The listing builds one solid part. Answer for the finished solid, in the listing's coordinates (mm). Face numbers are marked on the shaded views. A direction names the side the tool comes from. Give positions to 0.01 mm unless a question says otherwise; leave off trailing zeros. Write each loop counter-clockwise with the first axis right and the second up, starting at its lowest first coordinate (ties: lowest second). Pieces come first, ordered by that corner, then holes. Notation, with made-up numbers: M -7,-3 L 25,-3 A25 ccw 25,13 Z; hole C 12,28 d6. An arc over 180 degrees is marked long. Return JSON: item names as keys, results as strings.
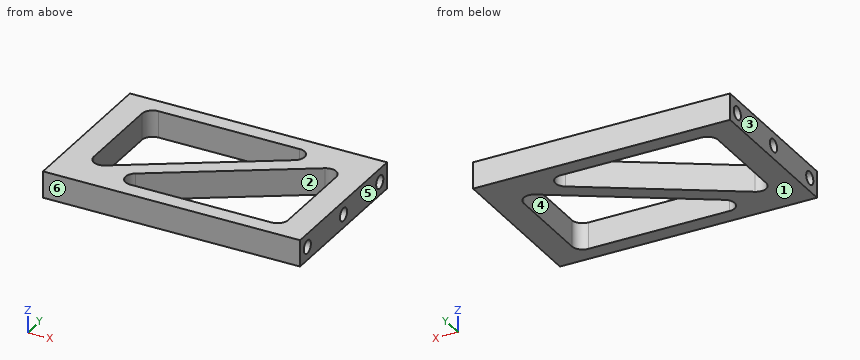
Autodesk Inventor part; units mm, degrees
ref_plane "YZ Plane" through (0, 0, 0) normal (1, 0, 0) x (0, 1, 0)
ref_plane "XZ Plane" through (0, 0, 0) normal (0, 1, 0) x (-1, 0, 0)
ref_plane "XY Plane" through (0, 0, 0) normal (0, 0, 1) x (1, 0, 0)
sketch "スケッチ1" plane through (0, 0, 0) normal (0, 0, 1) x (1, 0, 0)
  line L0 (-24.25, 15) -> (24.25, 15)
  line L1 (24.25, 15) -> (24.25, -15)
  line L2 (24.25, -15) -> (-24.25, -15)
  line L3 (-24.25, -15) -> (-24.25, 15)
  line L4 (-19.25, 12) -> (19.25, 12) construction
  line L5 (19.25, 12) -> (19.25, -12) construction
  line L6 (19.25, -12) -> (-19.25, -12) construction
  line L7 (-19.25, -12) -> (-19.25, 12) construction
  line L8 (19.25, 12) -> (-19.25, -12) construction
  line L9 (-19.25, -10.2324) -> (-19.25, 12)
  line L10 (-19.25, 12) -> (16.4145, 12)
  line L11 (16.4145, 12) -> (-19.25, -10.2324)
  line L12 (-16.4145, -12) -> (19.25, -12)
  line L13 (19.25, -12) -> (19.25, 10.2324)
  line L14 (19.25, 10.2324) -> (-16.4145, -12)
  line L15 (-24.25, 12.5) -> (24.25, 12.5) construction
  line L16 (24.25, -12.5) -> (-24.25, -12.5) construction
  line L17 (24.25, 12.5) -> (24.25, -12.5) construction
  point P0 (0, 0)
  point P1 (0, 12)
  point P2 (0, 15)
  point P3 (19.25, 0)
  point P4 (24.25, 0)
  dimension "d0" = 5
  dimension "d1" = 3
  dimension "d2" = 1.5
  dimension "d3" = 25
  dimension "d4" = 2.5
  dimension "d16" = 48.5
extrude "押し出し1" add sketch "スケッチ1" along normal blind 5
sketch "スケッチ2" plane through (24.25, -15, 0) normal (1, 0, 0) x (0, 0, -1)
  line L0 (0, 30) -> (-5, 30)
  line L1 (-5, 0) -> (-5, 30)
  line L2 (0, 15) -> (-5, 15) construction
  point P0 (-2.5, 2.5)
  point P1 (-2.5, 15)
  point P2 (-2.5, 27.5)
  point P3 (-2.5, 30)
  dimension "d7" = 25
hole "穴1" at (24.25, -12.5, 2.5) at (24.25, 0, 2.5) at (24.25, 12.5, 2.5) direction (-1, 0, 0) diameter 2.459 depth 3
mirror "ミラー1" about plane through (0, 0, 0) normal (1, 0, 0) of "穴1"
fillet "フィレット1" radius 2 6 edges at (-16.4145, -12, 2.5) (-19.25, -10.2324, 2.5) (19.25, 10.2324, 2.5) (19.25, -12, 2.5) (-19.25, 12, 2.5) (16.4145, 12, 2.5)
equation "\"d3\" = d5_1"
properties part number "リンク_ふともも_サブフレーム_1_2(予備案)" material "アルミニウム 2014-T4"
Item 1: A cutting plane is placed at A-A, the plane z = 4.4. Write down the section's boundary in (x, y), plus the area to 3 significant figures.
Geometry results:
{"outline": "M -24.25,-15 L 24.25,-15 L 24.25,15 L -24.25,15 Z; hole M -19.25,-6.63 A2 ccw -16.19,-8.33 L 10.48,8.3 A2 ccw 9.43,12 L -17.25,12 A2 ccw -19.25,10 Z; hole M -10.48,-8.3 A2 ccw -9.43,-12 L 17.25,-12 A2 ccw 19.25,-10 L 19.25,6.63 A2 ccw 16.19,8.33 Z", "area": "687 mm2"}
Item 2: Determine the mould class of the marked faces 3, 4, 5 and 6 for opening direction X: +X half, -X half, draft (parallel to the pull), parting line (faces both ways), or undercut.
Geometry results:
{"face 3": "-X half", "face 4": "undercut", "face 5": "+X half", "face 6": "draft"}
Item 3: Find the intervals of material crossed by line 1 (Y direction, x = 23.6, z = 2.5); line 2 (Z direction, x = -22.3, y = 12.5); line 3 (Y direction, x = 1, z = 3), in increasing order.
Geometry results:
{"line 1": "y = -15 to -13.73, -11.27 to -1.23, 1.23 to 11.27, 13.73 to 15", "line 2": "z = 0 to 1.27, 3.73 to 5", "line 3": "y = -15 to -12, -1.14 to 2.39, 12 to 15"}
Item 4: A cutting plane is placed at C-C, the plane y = 0. Write down the section's boundary in (x, z).
Geometry results:
{"outline": "M -24.25,0 L -19.25,0 L -19.25,5 L -24.25,5 L -24.25,3.73 L -21.25,3.73 L -21.25,1.27 L -24.25,1.27 Z; M -2.84,0 L 2.84,0 L 2.84,5 L -2.84,5 Z; M 19.25,0 L 24.25,0 L 24.25,1.27 L 21.25,1.27 L 21.25,3.73 L 24.25,3.73 L 24.25,5 L 19.25,5 Z"}
Item 5: Which of the six approach directions +Z, -Z, +X, -X, +Y, -Y give full straight-line access (tool end or side, diameter ignored) to the marked faces 1 and 2?
Geometry results:
{"face 1": "-Z, +X, -X, +Y, -Y", "face 2": "+Z, -Z"}
Item 6: Given pin 1 Ø1.2 at (y, z) = (-12.5, 2.5) entering from +X; pin 2 Ø1.5 at (y, z) = (12.5, 2.5) entering from -X, each flat-ended and moving along its own axis, determine where each tip first touches the part or whether it passes through.
Geometry results:
{"pin 1": "stops at x = 21.25", "pin 2": "stops at x = -21.25"}
Item 7: A cutting plane is placed at B-B, the plane x = 10. Write down the section's boundary in (y, z), plus the area to 3 significant figures.
Geometry results:
{"outline": "M -15,0 L -12,0 L -12,5 L -15,5 Z; M 4.47,0 L 8,0 L 8,5 L 4.47,5 Z; M 11.92,0 L 15,0 L 15,5 L 11.92,5 Z", "area": "48.1 mm2"}
Item 8: A cutting plane is placed at D-D, the plane y = -12.5. Write down the section's boundary in (x, z).
Geometry results:
{"outline": "M -24.25,0 L 24.25,0 L 24.25,1.27 L 21.25,1.27 L 21.25,3.73 L 24.25,3.73 L 24.25,5 L -24.25,5 L -24.25,3.73 L -21.25,3.73 L -21.25,1.27 L -24.25,1.27 Z"}
